Autodesk Inventor part; units mm, degrees
ref_plane "YZ Plane" through (0, 0, 0) normal (1, 0, 0) x (0, 1, 0)
ref_plane "XZ Plane" through (0, 0, 0) normal (0, 1, 0) x (-1, 0, 0)
ref_plane "XY Plane" through (0, 0, 0) normal (0, 0, 1) x (1, 0, 0)
sketch "Náčrt8" plane through (0, 0, 0) normal (0, 1, 0) x (-1, 0, 0)
  line L0 (-15, 15) -> (15, 15)
  line L1 (15, 15) -> (15, -15)
  line L2 (15, -15) -> (-15, -15)
  line L3 (-15, -15) -> (-15, 15)
  line L4 (-15, 15) -> (15, -15) construction
  line L5 (15, 15) -> (-15, -15) construction
  point P0 (0, 0)
  dimension "d67" = 30
  dimension "d68" = 30
extrude "Vysunutí8" add sketch "Náčrt8" along normal blind 30
sketch "Náčrt9" plane through (0, 30, 0) normal (0, 1, 0) x (1, 0, 0)
  line L0 (13, -13) -> (-13, -13)
  line L1 (-13, -13) -> (-13, 13)
  line L2 (-13, 13) -> (13, 13)
  line L3 (13, 13) -> (13, -13)
  line L4 (13, -13) -> (-13, 13) construction
  line L5 (-13, -13) -> (13, 13) construction
  point P0 (0, 0)
  dimension "d71" = 26
  dimension "d72" = 26
extrude "Vysunutí9" add sketch "Náčrt9" along normal blind 60
sketch "Náčrt10" plane through (-15, 0, -15) normal (-1, 0, 0) x (0, 0, 1)
  line L0 (30, 0) -> (0, 0)
  line L1 (30, 0) -> (30, 30)
  line L2 (0, 30) -> (30, 30)
  line L3 (0, 0) -> (0, 30)
  line L4 (28, 2) -> (2, 2)
  line L5 (2, 2) -> (2, 28)
  line L6 (2, 28) -> (28, 28)
  line L7 (28, 28) -> (28, 2)
  line L8 (28, 2) -> (2, 28) construction
  line L9 (2, 2) -> (28, 28) construction
  point P0 (15, 0)
  point P1 (7.5, 15)
  point P2 (15, 15)
  dimension "d79" = 26
  dimension "d80" = 26
  dimension "d120" = 15
  dimension "d121" = 15
sketch "Náčrt11" plane through (15, 0, -15) normal (0, 0, -1) x (-1, 0, 0)
  line L0 (30, 0) -> (0, 0)
  line L1 (30, 0) -> (30, 30)
  line L2 (0, 30) -> (30, 30)
  line L3 (0, 0) -> (0, 30)
  line L4 (28, 2) -> (2, 2)
  line L5 (2, 2) -> (2, 28)
  line L6 (2, 28) -> (28, 28)
  line L7 (28, 28) -> (28, 2)
  line L8 (28, 2) -> (2, 28) construction
  line L9 (2, 2) -> (28, 28) construction
  point P0 (15, 0)
  point P1 (15, 15)
  dimension "d87" = 26
  dimension "d88" = 26
  dimension "d122" = 15
  dimension "d123" = 15
sketch "Náčrt12" plane through (15, 0, 15) normal (1, 0, 0) x (0, 0, -1)
  line L0 (2, 2) -> (28, 2)
  line L1 (28, 28) -> (2, 28)
  line L2 (28, 2) -> (28, 28)
  line L3 (2, 28) -> (2, 2)
  point P0 (15, 0)
sketch "Náčrt13" plane through (0, 0, 0) normal (0, -1, 0) x (1, 0, 0)
  line L0 (13, -13) -> (13, 13)
  line L1 (-13, -13) -> (13, -13)
  line L2 (-15, 15) -> (15, 15)
  line L3 (13, 13) -> (-13, 13)
  line L4 (-13, 13) -> (-13, -13)
sketch "Náčrt14" plane through (-15, 0, 15) normal (0, 0, 1) x (1, 0, 0)
  line L0 (28, 28) -> (2, 28)
  line L1 (2, 28) -> (2, 2)
  line L2 (2, 2) -> (28, 2)
  line L3 (28, 2) -> (28, 28)
  point P0 (15, 0)
extrude "Vysunutí10" add sketch "Náčrt11" along normal blind 60 contours L4 L5 L6 L7
extrude "Vysunutí11" add sketch "Náčrt14" along normal blind 60
extrude "Vysunutí12" [suppressed]
extrude "Vysunutí13" [suppressed]
extrude "Vysunutí14" [suppressed]
chamfer "Zkosení13" [suppressed]
chamfer "Zkosení14" distance 2 angle 45 4 edges at (13, 15, -75) (-13, 15, -75) (0, 28, -75) (0, 2, -75)
chamfer "Zkosení15" [suppressed]
chamfer "Zkosení16" distance 2 angle 45 4 edges at (-13, 15, 75) (13, 15, 75) (0, 28, 75) (0, 2, 75)
chamfer "Zkosení17" distance 2 angle 45 4 edges at (-13, 90, 0) (0, 90, -13) (13, 90, 0) (0, 90, 13)
chamfer "Zkosení18" [suppressed]
equation "\"d67\" = width"
equation "\"d68\" = width"
equation "\"d69\" = width"
equation "\"d71\" = width - 2 * thickness"
equation "\"d72\" = width - 2 * thickness"
equation "\"d75\" = 2 * width"
equation "\"d79\" = width - 2 * thickness"
equation "\"d80\" = width - 2 * thickness"
equation "\"d87\" = width - 2 * thickness"
equation "\"d88\" = width - 2 * thickness"
equation "\"d89\" = 2 * width"
equation "\"d91\" = 2 * width"
equation "\"d93\" = 2 * width"
equation "\"d95\" = 2 * width"
equation "\"d97\" = 2 * width"
equation "\"d99\" = thickness"
equation "\"d102\" = thickness"
equation "\"d105\" = thickness"
equation "\"d108\" = thickness"
equation "\"d111\" = thickness"
equation "\"d114\" = thickness"
equation "\"width\" = 30"
equation "\"thickness\" = 2"
properties part number "Profile-Connector#04" material "PVC potrubí"
The model under review builds one solid part; all positions refer to its coordinate system, in mm. A direction names the side the tool comes from. Coordinates: 2 decimals unless noted, no trailing zeros. Write each loop counter-clockwise with the first axis right and the second up, starting at its lowest first coordinate (ties: lowest second). Pieces come first, ordered by that corner, then holes.
1) We need section D-D on y = 66.5. State the section outline as (x, z) points, then the cut area to 3 significant figures.
2) We need section C-C on z = -9. State the section outline as (x, y) points.
3) We need section B-B on x = -6.75. State the section outline as (y, z) points, then the cut area to 3 significant figures.
4) To check wall thickness, follow probe 1 along Z at (x, y) = (3.5, 78); probe 2 along Y at (x, z) = (2, -61.5). State the ranges of each line that lie inside material, in increasing order.
5) Machinability: for faces 1 (the face through (-13, 15, 44)), 2 (the face through (-13, 15, -44)), 3 (the face through (13, 59, 0)), which of the approach directions +Z, -Z, +X, -X, +Y, -Y give a long, thin tool a straight path to every point of the face, cutting with its end or side? Answer none if there is none.
6) Clearance check with flat-ended pins moving along their axes: pin 1 Ø12 at (x, z) = (-12, -22) entering from +Y; pin 2 Ø21 at (y, z) = (67.5, 1) entering from +X; pin 3 Ø8 at (y, z) = (12.5, -36.5) entering from -X; pin 4 Ø8 at (x, z) = (-4, 16.5) entering from -Y. State where each tip first meets the part, or that it passes through.
7) We need section A-A on y = 16. State the section outline as (x, z) points.
Answer list:
1. outline: (-13, -13) - (13, -13) - (13, 13) - (-13, 13) - close
1. area: 676 mm2
2. outline: (-15, 0) - (15, 0) - (15, 30) - (13, 30) - (13, 88) - (11, 90) - (-11, 90) - (-13, 88) - (-13, 30) - (-15, 30) - close
3. outline: (0, -15) - (2, -15) - (2, -73) - (4, -75) - (26, -75) - (28, -73) - (28, -15) - (30, -15) - (30, -13) - (88, -13) - (90, -11) - (90, 11) - (88, 13) - (30, 13) - (30, 15) - (28, 15) - (28, 73) - (26, 75) - (4, 75) - (2, 73) - (2, 15) - (0, 15) - close
3. area: 5,570 mm2
4. probe 1: z = -13 to 13
4. probe 2: y = 2 to 28
5. face 1: +Z, -X, +Y, -Y
5. face 2: -Z, -X, +Y, -Y
5. face 3: +Z, -Z, +X, +Y
6. pin 1: stops at y = 28
6. pin 2: stops at x = 13
6. pin 3: stops at x = -13
6. pin 4: stops at y = 0
7. outline: (-15, -15) - (-13, -15) - (-13, -73) - (-11, -75) - (11, -75) - (13, -73) - (13, -15) - (15, -15) - (15, 15) - (13, 15) - (13, 73) - (11, 75) - (-11, 75) - (-13, 73) - (-13, 15) - (-15, 15) - close
